Answer from the drawing. Dimensions are ordinates in mm from the lowest x, y and z of the part. Round coordinates to 2 decimals unless told otherwise and drop trailing zeros. Loops run counter-clockwise (first coordinate to the right, second up) from the corner with the lowest first, then second, coordinate; pieces in that order, holes last. Notation, with made-up numbers: M 72.25,-34.75 L 112.25,-34.75 A22 ccw 112.25,-1.75 Z; hole C 73,10 d5. An arc over 180 degrees is marked long. Answer as a JSON object with one key per item and string values.
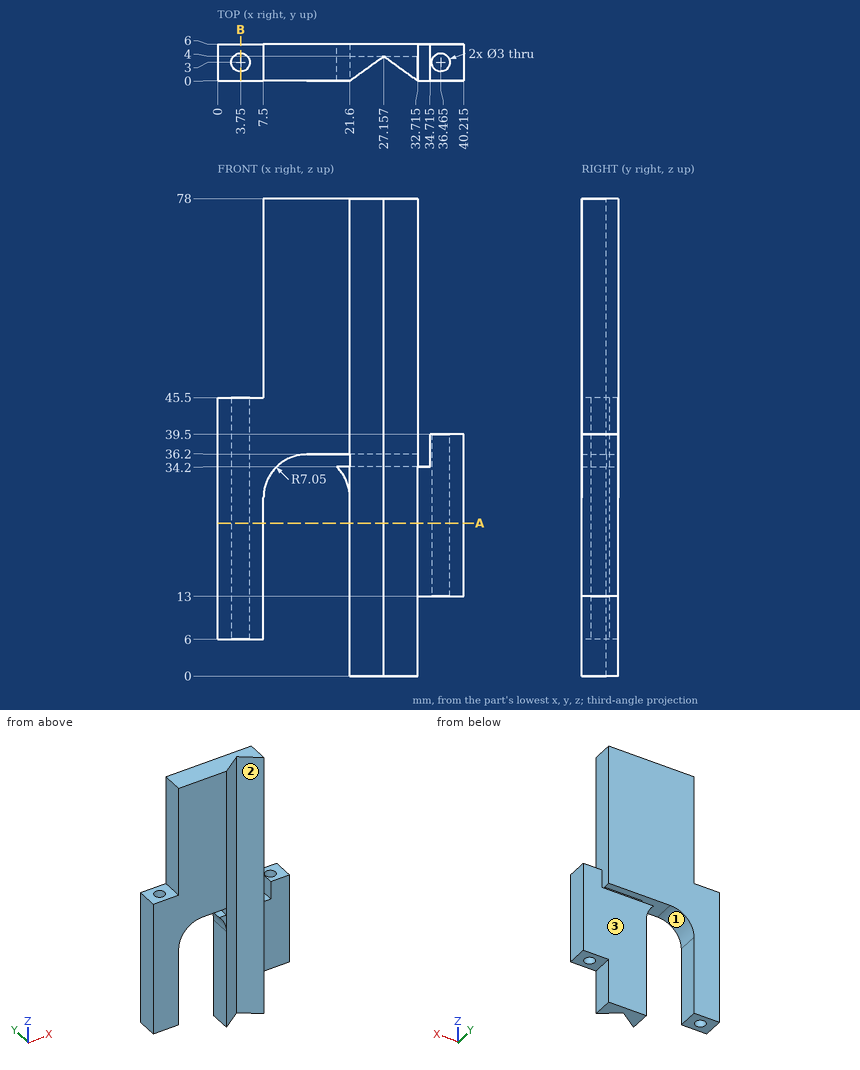
Item 1: The part is cut by section B-B (x = 3.75). Give the vertices of the cut face in (y, z).
Values follow:
{"outline": "M 0,6 L 1.5,6 L 1.5,45.5 L 0,45.5 Z; M 4.5,6 L 6,6 L 6,45.5 L 4.5,45.5 Z"}
Item 2: The part is cut by section A-A (z = 25). Give the number of separate pieces and of enclosed holes in the cut face, then the cut area to 3 significant figures.
Values follow:
{"separate pieces": "2", "enclosed holes": "2", "area": "120 mm^2"}
Item 3: Determine the mould class of the marked faces 1, 2 and 3 for opening direction X: released by +X, released by -X, zero draft, split by the parting line, or undercut.
Values follow:
{"face 1": "undercut", "face 2": "undercut", "face 3": "zero draft"}
Item 4: Straight lines are drawn through the part: line 1 (Z direction, x = 29.5, y = 5.5); line 2 (Y direction, x = 3.75, z = 37); line 3 (X direction, y = 1.15, z = 10.5) (1 decimal). For each, find the intervals that lie inside material, in ascending order.
Values follow:
{"line 1": "0 to 34.2, 36.2 to 78", "line 2": "0 to 1.5, 4.5 to 6", "line 3": "0 to 7.5, 21.6 to 23.2, 31.1 to 32.7"}
Item 5: Flat-ended cylindrical pins translate along their axes: P1, Ø2, axis at y = 1.5, z = 58.5, coming from the -X side; P2, Ø1.8, axis at y = 3, z = 49.5, coming from the +X side (1 decimal); P3, Ø1.8, axis at x = 36, y = 2, coming from the -Z side; P4, Ø2, axis at x = 9, z = 26, coming from the +Y side. Find the tip coordinate at first contact, or state that the pin passes through.
Values follow:
{"P1": "x = 7.5", "P2": "x = 32.7", "P3": "z = 13", "P4": "through"}
